from build123d import *

# Parameters (mm, degrees)
F0_W     = 38.1
F0_H     = 19.05
F0_H_2   = 12.7
F0_W_2   = 19.05
F1_DEPTH = 19.05
F3_DEPTH = 19.05
F5_DEPTH = 19.05
F7_START = -6.35
F6_R     = 12.7
F6_R_2   = 11.1125
F7_DEPTH = 6.35
F8_DEPTH = 50.801


with BuildPart() as f1:
    # F0 (on Front) → F1 (new body, symmetric)
    with BuildSketch(Plane.XZ):
        with Locations((0, 41.275)):
            Rectangle(F0_W, F0_H)
        with Locations((0, 25.4)):
            Rectangle(F0_W, F0_H_2)
        with Locations((0, 9.525)):
            Rectangle(F0_W, F0_H)
        with Locations((-28.575, 25.4)):
            Rectangle(F0_W_2, F0_H_2)
        with Locations((28.575, 25.4)):
            Rectangle(F0_W_2, F0_H_2)
    extrude(amount=F1_DEPTH, both=True)

    # F2 (on face) → F3 (cut)
    with BuildSketch(Plane.XY.offset(50.8)):
        with BuildLine():
            ThreePointArc((-19.05, 0), (-13.4703841816, 13.4703841816), (0, 19.05))
            Line((0, 19.05), (-19.05, 19.05))
            Line((-19.05, 19.05), (-19.05, 0))
        make_face()
        with BuildLine():
            ThreePointArc((0, 19.05), (13.4703841816, 13.4703841816), (19.05, 0))
            Line((19.05, 0), (19.05, 19.05))
            Line((19.05, 19.05), (0, 19.05))
        make_face()
        with BuildLine():
            Line((-19.05, -19.05), (-3.68e-08, -19.05))
            ThreePointArc((-3.68e-08, -19.05), (-13.4703841946, -13.4703841686), (-19.05, 0))
            Line((-19.05, 0), (-19.05, -19.05))
        make_face()
        with BuildLine():
            Line((19.05, -19.05), (19.05, 0))
            ThreePointArc((19.05, 0), (13.4703841686, -13.4703841946), (-3.68e-08, -19.05))
            Line((-3.68e-08, -19.05), (19.05, -19.05))
        make_face()
    extrude(amount=-F3_DEPTH, mode=Mode.SUBTRACT)

    # F4 (on face) → F5 (cut)
    with BuildSketch(Plane(origin=(0, 0, 0), x_dir=(1, 0, 0), z_dir=(0, 0, -1))):
        with BuildLine():
            ThreePointArc((-19.05, -3.68e-08), (-13.4703841946, 13.4703841686), (0, 19.05))
            Line((0, 19.05), (-19.05, 19.05))
            Line((-19.05, 19.05), (-19.05, -3.68e-08))
        make_face()
        with BuildLine():
            ThreePointArc((0, 19.05), (13.4703841816, 13.4703841816), (19.05, 0))
            Line((19.05, 0), (19.05, 19.05))
            Line((19.05, 19.05), (0, 19.05))
        make_face()
        with BuildLine():
            Line((19.05, -19.05), (19.05, 0))
            ThreePointArc((19.05, 0), (13.4703841686, -13.4703841946), (-3.68e-08, -19.05))
            Line((-3.68e-08, -19.05), (19.05, -19.05))
        make_face()
        with BuildLine():
            Line((-19.05, -19.05), (-3.68e-08, -19.05))
            ThreePointArc((-3.68e-08, -19.05), (-13.4703841816, -13.4703841816), (-19.05, -3.68e-08))
            Line((-19.05, -3.68e-08), (-19.05, -19.05))
        make_face()
    extrude(amount=-F5_DEPTH, mode=Mode.SUBTRACT)

    # F6 (on face) → F7 (cut)
    with BuildSketch(Plane.XY.offset(50.8).offset(F7_START)):
        Circle(F6_R)
        Circle(F6_R_2, mode=Mode.SUBTRACT)
    extrude(amount=-F7_DEPTH, mode=Mode.SUBTRACT)

    # F6 (on face) → F8 (cut, through all)
    with BuildSketch(Plane.XY.offset(50.8)):
        Circle(F6_R_2)
    extrude(amount=-F8_DEPTH, mode=Mode.SUBTRACT)


solid = f1.part
Could you check a few things on this model? Use its own coordinates, in mm. A direction names the side the tool comes from. Round coordinates to 2 decimals unless told otherwise and drop trailing zeros. Order: outer loops, then holes, each group sorted by start corner. A loop starts at its lowest first (then second) coordinate and runs counter-clockwise, first axis right, second up.
(1) Which directions (+Z, -Z, +X, -X, +Y, -Y) give clear straight access to the entire face, cutting with the end or side of a thin tool? Please do faces 4 (the flat face through (27, 0, 31.75)), 5 (the flat face through (27, 0, 19.05)), 6 (the flat face through (-1, 19.05, 25)), 7 (the flat face through (0.88, -11.23, 44.45)).
Response values:
face 4: +Z, +X
face 5: -Z, +X
face 6: +Z, -Z, +X, -X, +Y
face 7: none
(2) Imagine slicing it at B-B (y = 1). Write out the boundary of the cut face in (x, z).
Response values:
outline: (-38.1, 19.05) - (-19.02, 19.05) - (-19.02, 0) - (-11.07, 0) - (-11.07, 38.1) - (-12.66, 38.1) - (-12.66, 44.45) - (-11.07, 44.45) - (-11.07, 50.8) - (-19.02, 50.8) - (-19.02, 31.75) - (-38.1, 31.75) - close; (11.07, 0) - (19.02, 0) - (19.02, 19.05) - (38.1, 19.05) - (38.1, 31.75) - (19.02, 31.75) - (19.02, 50.8) - (11.07, 50.8) - (11.07, 44.45) - (12.66, 44.45) - (12.66, 38.1) - (11.07, 38.1) - close
(3) If we mould it in two halves opening along Y, with no side actions, what happens to faces 1 (the flat face through (-1, -19.05, 25)), 2 (the flat face through (-28, 0, 31.75)), 3 (the cylindrical face through (10.6, 3.34, 47.67))? For each: released by +Y, released by -Y, zero draft, split by the parting line, or undercut.
Response values:
face 1: released by -Y
face 2: zero draft
face 3: undercut
(4) Please list where these lines run through material, in increasing order: line 1 along Y through (x, z) = (0, 46.5); line 2 along Y through (x, z) = (0, 39.5); line 3 along X through (y, z) = (0.5, 34.5).
Response values:
line 1: y = -19.05 to -11.11, 11.11 to 19.05
line 2: y = -19.05 to -12.7, 12.7 to 19.05
line 3: x = -19.04 to -11.1, 11.1 to 19.04
(5) Imagine slicing it at D-D (x = -16.5). Write out the boundary of the cut face in (y, z), plus the area to 3 significant figures.
Response values:
outline: (-19.05, 19.05) - (-9.52, 19.05) - (-9.52, 0) - (9.52, 0) - (9.52, 19.05) - (19.05, 19.05) - (19.05, 31.75) - (9.52, 31.75) - (9.52, 50.8) - (-9.52, 50.8) - (-9.52, 31.75) - (-19.05, 31.75) - close
area: 1,210 mm2
(6) I'm going to push flat-ended pins straight in: pin 1 (6 mm diameter, centred on x = 5, y = 2.5, fed in from +Z); pin 2 (12 mm diameter, centred on x = 17, y = -14, fed in from +Z); pin 3 (4 mm diameter, centred on y = 7, z = 36.5, fed in from -X); pin 4 (1.5 mm diameter, centred on x = -10, z = 11.5, fed in from -Y). Where does each tip first touch, or does it pass through?
Response values:
pin 1: passes through
pin 2: stops at z = 50.8
pin 3: stops at x = -18.38
pin 4: stops at y = -16.65
(7) Imagine slicing it at C-C (z = 40). Write out the boundary of the cut face in (x, y).
Response values:
outline: circle Ø38.1 at (0, 0); hole circle Ø25.4 at (0, 0)
